Here's how the part is built. I have some questions about the finished solid (model axes, mm). A direction names the side the tool comes from. Round coordinates to 2 decimals unless told otherwise and drop trailing zeros. Order: outer loops, then holes, each group sorted by start corner. A loop starts at its lowest first (then second) coordinate and runs counter-clockwise, first axis right, second up. Notation, with made-up numbers: (40.25, 44.5) -> (72.25, 44.5) arc R10 ccw to (72.25, 61.5) -> close; hole circle Ø5 at (39.25, -31). An arc over 180 degrees is marked (long way). Use a Markdown table: item, result. Add a question column.
(1) I want a section at B-B, the plane y = -41. Please give me the cut outline in (x, z).
(2) If I drill on probe 1 along Y at (x, z) = (-31, 0.3); probe 2 along X at (y, z) = (15.5, 0); probe 3 along Y at (x, z) = (-29, -1.35), over which ranges is the centre line in solid material (lowest first)?
(3) I want a section at A-A, the plane x = 0. Please give me the cut outline in (y, z), then the cut area to 3 significant figures.
(4) I'm going to push flat-ended pins straight in: P1, Ø1.5, axis at x = -16.5, z = 1, coming from the -Y side; P2, Ø1.6, axis at y = -3.5, z = 0, coming from the -X side; P3, Ø1, axis at y = 12.5, z = -2, coming from the +X side. Where does each tip first touch, or does it pass through?
(5) On a 3-axis mill with a long thin cutter (end or side, diameter ignored), from which of +Z, -Z, +X, -X, +Y, -Y can I reach the whole of each face in a straight line? I mean faces 1 (the face through (59, -46, 0.598)), 2 (the face through (-32, -4, 0)), 3 (the face through (-45, -5, 0)), 4 (the face through (-8.34, 18.89, 0.04)). Say none if no direction works.
(6) I want a section at C-C, the plane z = -0.4. Give the number of separate pieces and of enclosed holes in the cut face, then the cut area to 3 significant figures.
(7) I want a section at D-D, the plane y = 6. Please give me the cut outline in (x, z).
(8) Thinking about a two-plate mould opening in X: for faces 5 (the face through (15.592, -20, 0)), 6 (the face through (1, -36, 0)), 7 (the face through (63.5, -42, 1)), 8 (the face through (-63.5, -42, 1)), which applies, pulls with the +X half, pulls with the -X half, needs draft (parallel to the pull), parting line crosses it, or undercut?
from build123d import *

# Parameters (mm, degrees)
PAD005005_DEPTH      = 2.5
SKETCH014_W          = 4
SKETCH014_H          = 2
POCKET003_DEPTH      = 298.676624
POCKET003_DEPTH_BACK = 298.676624
POCKET004_DEPTH      = 2.501
POCKET004_DEPTH_BACK = 2.501
POCKET005_DEPTH      = 2.501
POCKET005_DEPTH_BACK = 2.501
SKETCH017_W          = 10.816708
SKETCH017_H          = 3.71916
POCKET006_DEPTH      = 312.676624


with BuildPart() as part:
    # Sketch013 → Pad005005 (new body, symmetric)
    with BuildSketch(Plane.XY):
        Polygon((-45, 0), (-15, 0), (-15, 12), (-45, 12), (-45, 22), (45, 22), (45, 12), (15, 12), (15, 0), (45, 0), (45, -10), (63.5, -34), (63.5, -54), (53.5, -54), (53.5, -36), (-53.5, -36), (-53.5, -54), (-63.5, -54), (-63.5, -34), (-45, -10), align=None)
    extrude(amount=PAD005005_DEPTH, both=True)

    # Sketch014 → Pocket003 (cut, two sides)
    with BuildSketch(Plane.XY) as pocket003_sk:
        with Locations((-32, -3)):
            Rectangle(SKETCH014_W, SKETCH014_H)
        with Locations((-32, 15)):
            Rectangle(SKETCH014_W, SKETCH014_H)
        with Locations((-23, -3)):
            Rectangle(SKETCH014_W, SKETCH014_H)
        with Locations((-23, 15)):
            Rectangle(SKETCH014_W, SKETCH014_H)
    pocket003 = extrude(amount=-POCKET003_DEPTH, mode=Mode.SUBTRACT) + extrude(pocket003_sk.sketch, amount=POCKET003_DEPTH_BACK, mode=Mode.SUBTRACT)

    # Mirrored002: Pocket003 across Sketch014 V_Axis
    add(pocket003.mirror(Plane(origin=(0, 0, 0), x_dir=(0, 0, 1), z_dir=(1, 0, 0))), mode=Mode.SUBTRACT)

    # Sketch015 → Pocket004 (cut, two sides)
    with BuildSketch(Plane.XY) as pocket004_sk:
        Polygon((-11.314059, 23.254717), (-6.157998, 15.686502), (6.157998, 15.686502), (11.314059, 23.254717), align=None)
    extrude(amount=-POCKET004_DEPTH, mode=Mode.SUBTRACT)
    extrude(pocket004_sk.sketch, amount=POCKET004_DEPTH_BACK, mode=Mode.SUBTRACT)

    # Sketch016 → Pocket005 (cut, two sides)
    with BuildSketch(Plane.XY) as pocket005_sk:
        Polygon((-7.975373, -5.942453), (-15.591735, -13.506808), (-15.591735, -25.932104), (15.591735, -25.932104), (15.591735, -13.506808), (7.975373, -5.942453), align=None)
    extrude(amount=-POCKET005_DEPTH, mode=Mode.SUBTRACT)
    extrude(pocket005_sk.sketch, amount=POCKET005_DEPTH_BACK, mode=Mode.SUBTRACT)

    # Sketch017 → Pocket006 (cut, through all)
    with BuildSketch(Plane.XZ.offset(37.5)):
        with Locations((-58.423876, -1.261529)):
            Rectangle(SKETCH017_W, SKETCH017_H)
    pocket006 = extrude(amount=POCKET006_DEPTH, mode=Mode.SUBTRACT)

    # Mirrored003: Pocket006 across Sketch017 V_Axis
    add(pocket006.mirror(Plane(origin=(0, -37.5, 0), x_dir=(0, -1, 0), z_dir=(1, 0, 0))), mode=Mode.SUBTRACT)


solid = part.part
Taken from the geometry:
| question | item | result |
|---|---|---|
| 1 | outline | (-63.5, 0.6) -> (-53.5, 0.6) -> (-53.5, 2.5) -> (-63.5, 2.5) -> close; (53.5, 0.6) -> (63.5, 0.6) -> (63.5, 2.5) -> (53.5, 2.5) -> close |
| 2 | probe 1 | y = -36 to -4, -2 to 0, 12 to 14, 16 to 22 |
| 2 | probe 2 | x = -45 to -34, -30 to -25, -21 to 21, 25 to 30, 34 to 45 |
| 2 | probe 3 | y = -36 to 0, 12 to 22 |
| 3 | outline | (-36, -2.5) -> (-25.93, -2.5) -> (-25.93, 2.5) -> (-36, 2.5) -> close; (-5.94, -2.5) -> (15.69, -2.5) -> (15.69, 2.5) -> (-5.94, 2.5) -> close |
| 3 | area | 158 mm2 |
| 4 | P1 | stops at y = -36 |
| 4 | P2 | stops at x = -45 |
| 4 | P3 | stops at x = 45 |
| 5 | face 1 | -Z, +X, -X, -Y |
| 5 | face 2 | +Z, -Z |
| 5 | face 3 | +Z, -Z, -X, +Y |
| 5 | face 4 | +Z, -Z, +Y |
| 6 | separate pieces | 1 |
| 6 | enclosed holes | 9 |
| 6 | area | 4,310 mm2 |
| 7 | outline | (-15, -2.5) -> (15, -2.5) -> (15, 2.5) -> (-15, 2.5) -> close |
| 8 | face 5 | undercut |
| 8 | face 6 | undercut |
| 8 | face 7 | pulls with the +X half |
| 8 | face 8 | pulls with the -X half |
